The drawing under review shows one solid part. Ordinate dimensions are in mm from its lowest x, y, z. A direction names the side the tool comes from. Coordinates: 2 decimals unless noted, no trailing zeros. Loops run counter-clockwise (first coordinate to the right, second up) from the corner with the lowest first, then second, coordinate; pieces in that order, holes last. Notation, with made-up numbers: M -10.5,-30 L 40.5,-30 A25 cw 40.5,-16 Z; hole C 16.25,27.25 d2. An arc over 180 degrees is marked long. Answer as a JSON object with one key per item and string values. Group by question number.
1. Draft analysis for pull direction Y (two halves, no side actions). For the marked faces 3, 4 and 5, state which applies: +Y half, -Y half, draft (parallel to the pull), parting line (faces both ways), or undercut.
2. Consider section C-C (z = 2.15). State the section outline as (x, y) points (1 decimal).
3. Insertion check: pin 1 (1.1 mm diameter, centred on x = 7, z = 1.5, fed in from +Y); pin 2 (2 mm diameter, centred on y = 10.5, z = 3, fed in from +X) (1 decimal); pin 3 (1.5 mm diameter, centred on x = 3.5, y = 3, fed in from -Z); pin 4 (1 mm diameter, centred on y = 2.5, z = 1.5, fed in from -X). Each pin has a flat end and moves straight along its axis. Give the tip position at first contact, or say it passes through.
4. Consider section D-D (y = 15.25). State the section outline as (x, z) points.
5. Machinability: for the marked faces 1 and 2, which of the approach directions +Z, -Z, +X, -X, +Y, -Y give a long, thin tool a straight path to every point of the face, cutting with its end or side? Answer none if there is none.
6. Consider section B-B (x = 10). State the section outline as (y, z) points (1 decimal).
7. To check wall thickness, follow probe 1 along X at (y, z) = (5.5, 3.25) (1 decimal); probe 2 along Y at (x, z) = (5.75, 0.7) (1 decimal); probe 3 along X at (y, z) = (6.25, 1.4) (1 decimal). State the ranges of each line that lie inside material, in increasing order.
8. Consider section A-A (y = 10.25). State the section outline as (x, z) points (1 decimal).
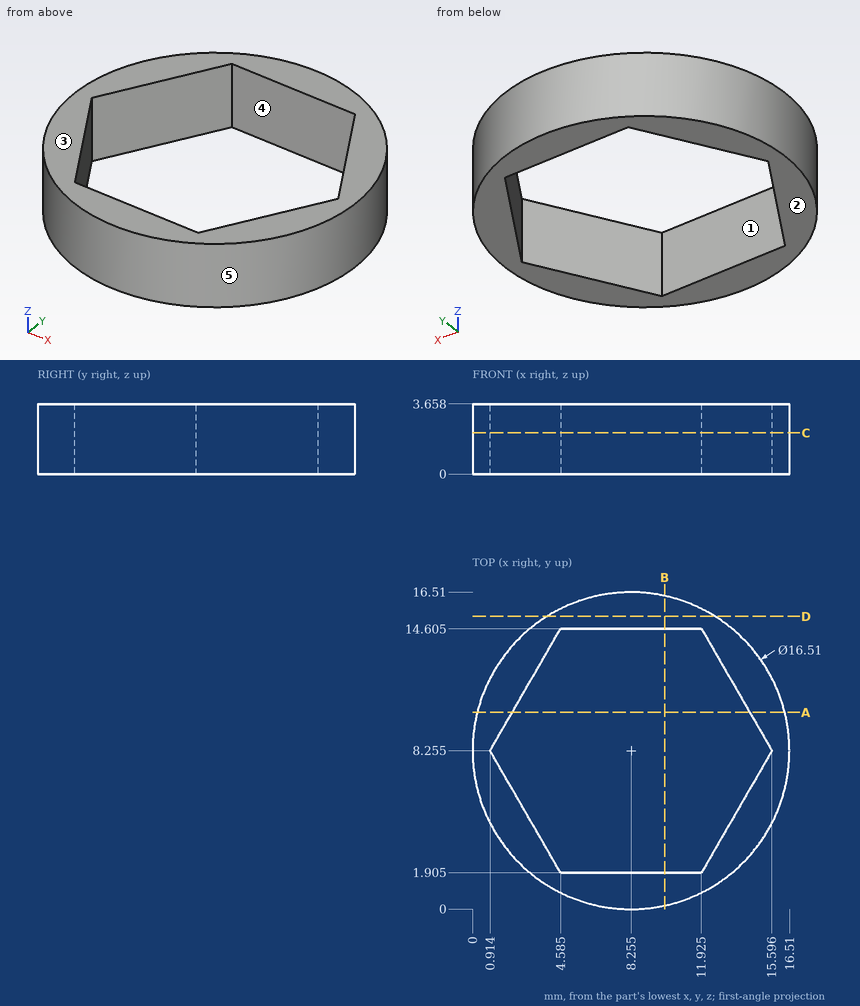
Findings below:
{
 "1": {"face 3": "draft", "face 4": "undercut", "face 5": "parting line"},
 "2": {"outline": "C 8.3,8.3 d16.5; hole M 0.9,8.3 L 4.6,1.9 L 11.9,1.9 L 15.6,8.3 L 11.9,14.6 L 4.6,14.6 Z"},
 "3": {"pin 1": "stops at y = 16.48", "pin 2": "stops at x = 16.4", "pin 3": "stops at z = 0", "pin 4": "stops at x = 1.89"},
 "4": {"outline": "M 3.87,0 L 12.64,0 L 12.64,3.66 L 3.87,3.66 Z"},
 "5": {"face 1": "+Z, -Z", "face 2": "-Z, +X, -X, +Y, -Y"},
 "6": {"outline": "M 0.2,0 L 1.9,0 L 1.9,3.7 L 0.2,3.7 Z; M 14.6,0 L 16.3,0 L 16.3,3.7 L 14.6,3.7 Z"},
 "7": {"probe 1": "x = 0.5 to 2.5, 14 to 16", "probe 2": "y = 0.4 to 1.9, 14.6 to 16.1", "probe 3": "x = 0.2 to 2.1, 14.4 to 16.3"},
 "8": {"outline": "M 0.2,0 L 2.1,0 L 2.1,3.7 L 0.2,3.7 Z; M 14.4,0 L 16.3,0 L 16.3,3.7 L 14.4,3.7 Z"}
}
